```python
from build123d import *

# Parameters (mm, degrees)
ESQUISSE1_R        = 2.5
ESQUISSE1_R_2      = 5
ESQUISSE1_R_3      = 8
BOSS_EXTRU_1_DEPTH = 6


with BuildPart() as part:
    # Esquisse1 → Boss.-Extru.1 (new body)
    with BuildSketch(Plane.XY):
        Polygon((0, 0), (200, 0), (200, 200), (150, 200), (150, 206), (100, 206), (100, 200), (50, 200), (50, 206), (0, 206), align=None)
        with Locations((175, 170)):
            Circle(ESQUISSE1_R, mode=Mode.SUBTRACT)
        with Locations((175, 160)):
            Circle(ESQUISSE1_R, mode=Mode.SUBTRACT)
        with Locations((25, 170)):
            Circle(ESQUISSE1_R, mode=Mode.SUBTRACT)
        with Locations((25, 160)):
            Circle(ESQUISSE1_R, mode=Mode.SUBTRACT)
        with Locations((120, 170)):
            Circle(ESQUISSE1_R_2, mode=Mode.SUBTRACT)
        with Locations((87, 47.14998282)):
            Circle(ESQUISSE1_R_3, mode=Mode.SUBTRACT)
        with Locations((113, 47.14998282)):
            Circle(ESQUISSE1_R_3, mode=Mode.SUBTRACT)
    extrude(amount=BOSS_EXTRU_1_DEPTH)


solid = part.part
```
Check sheet for the modelled part. Datum: model origin and axes. Units: mm. A direction names the side the tool comes from. Round coordinates to 2 decimals unless told otherwise and drop trailing zeros. Loops run counter-clockwise (first coordinate to the right, second up) from the corner with the lowest first, then second, coordinate; pieces in that order, holes last. Notation, with made-up numbers: (79, -9) -> (100, -9) arc R33 cw to (100, 30) -> close; hole circle Ø4 at (30, 9). An arc over 180 degrees is marked (long way). Answer in a Markdown table with one row per item.
Q1. Sectioned sample at D-D on z = 2.85. Enter the section's corners in (x, y).
Data:
| item | result |
|---|---|
| outline | (0, 0) -> (200, 0) -> (200, 200) -> (150, 200) -> (150, 206) -> (100, 206) -> (100, 200) -> (50, 200) -> (50, 206) -> (0, 206) -> close; hole circle Ø5 at (25, 160); hole circle Ø5 at (25, 170); hole circle Ø16 at (87, 47.15); hole circle Ø16 at (113, 47.15); hole circle Ø10 at (120, 170); hole circle Ø5 at (175, 160); hole circle Ø5 at (175, 170) |
Q2. Sectioned sample at A-A on y = 160. Enter the section's corners in (x, z).
Data:
| item | result |
|---|---|
| outline | (0, 0) -> (22.5, 0) -> (22.5, 6) -> (0, 6) -> close; (27.5, 0) -> (172.5, 0) -> (172.5, 6) -> (27.5, 6) -> close; (177.5, 0) -> (200, 0) -> (200, 6) -> (177.5, 6) -> close |
Q3. Release check for a two-part mould opening along X. For faces 1 (the face through (24.67, 162.48, 2.96)), 2 (the face through (0, 104, 3)), 3 (the face through (200, 99, 3)), 4 (the face through (99, 104, 6)) record: released by +X, released by -X, zero draft, split by the parting line, or undercut.
Data:
| item | result |
|---|---|
| face 1 | undercut |
| face 2 | released by -X |
| face 3 | released by +X |
| face 4 | zero draft |
Q4. Sectioned sample at B-B on x = 175. Enter the section's corners in (y, z).
Data:
| item | result |
|---|---|
| outline | (0, 0) -> (157.5, 0) -> (157.5, 6) -> (0, 6) -> close; (162.5, 0) -> (167.5, 0) -> (167.5, 6) -> (162.5, 6) -> close; (172.5, 0) -> (200, 0) -> (200, 6) -> (172.5, 6) -> close |
Q5. Sectioned sample at C-C on x = 87. Enter the section's corners in (y, z), then the cut area to 3 significant figures.
Data:
| item | result |
|---|---|
| outline | (0, 0) -> (39.15, 0) -> (39.15, 6) -> (0, 6) -> close; (55.15, 0) -> (200, 0) -> (200, 6) -> (55.15, 6) -> close |
| area | 1,100 mm^2 |
Q6. Go/stop test with flat-tipped pins: P1, Ø1.8, axis at x = 167.5, z = 4.5, coming from the +Y side; P2, Ø9.5, axis at x = 113, y = 47.15, coming from the -Z side; P3, Ø1.8, axis at y = 202, z = 4, coming from the +X side. Record where each tip stops, or that it passes through.
Data:
| item | result |
|---|---|
| P1 | stops at y = 200 |
| P2 | passes through |
| P3 | stops at x = 150 |
Q7. Set-up check for faces 5 (the face through (150, 203, 3)), 6 (the face through (25, 206, 3)), 7 (the face through (50, 203, 3)): record each of +Z, -Z, +X, -X, +Y, -Y from which the full face is reachable in a straight line by a thin tool's end or side.
Data:
| item | result |
|---|---|
| face 5 | +Z, -Z, +X, +Y |
| face 6 | +Z, -Z, +X, -X, +Y |
| face 7 | +Z, -Z, +Y |
Q8. Thickness scan on L1, parallel to Y at x = 175, z = 3.2; L2, parallel to Y at x = 25, z = 3.7; L3, parallel to X at y = 47, z = 5.05. Record the ranges inside material, lowest first.
Data:
| item | result |
|---|---|
| L1 | y = 0 to 157.5, 162.5 to 167.5, 172.5 to 200 |
| L2 | y = 0 to 157.5, 162.5 to 167.5, 172.5 to 206 |
| L3 | x = 0 to 79, 95 to 105, 121 to 200 |
